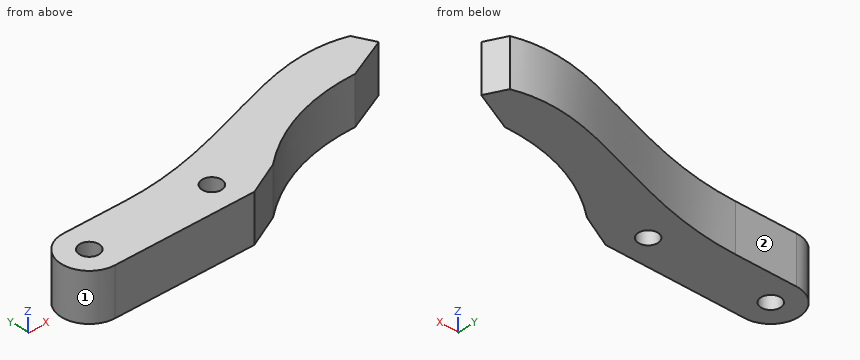
from build123d import *

# Parameters (mm, degrees)
SKETCH1_R           = 5
SKETCH1_R_2         = 1.75
BOSS_EXTRUDE1_DEPTH = 8.5
BOSS_EXTRUDE2_START = -8.5
BOSS_EXTRUDE2_DEPTH = 8.5


with BuildPart() as part:
    # Sketch1 → Boss-Extrude1 (new body)
    # profile 1 of 3: a face of its own
    with BuildSketch(Plane.XY):
        with Locations((-11, 0)):
            Circle(SKETCH1_R)
        with Locations((-11, 0)):
            Circle(SKETCH1_R_2, mode=Mode.SUBTRACT)
    # profile 2 of 3: a face of its own
    with BuildSketch(Plane.XY):
        with BuildLine():
            Line((11, 5), (-11, 5))
            ThreePointArc((-11, 5), (-7.464466094, 3.535533906), (-6, 0))
            ThreePointArc((-6, 0), (-7.464466094, -3.535533906), (-11, -5))
            Line((-11, -5), (11, -5))
            ThreePointArc((11, -5), (6, 0), (11, 5))
        make_face()
    # profile 3 of 3: a face of its own
    with BuildSketch(Plane.XY):
        with Locations((11, 0)):
            Circle(SKETCH1_R)
        with Locations((11, 0)):
            Circle(SKETCH1_R_2, mode=Mode.SUBTRACT)
    extrude(amount=BOSS_EXTRUDE1_DEPTH)

    # Sketch2 → Boss-Extrude2 (add)
    with BuildSketch(Plane.XY.offset(8.5).offset(BOSS_EXTRUDE2_START)):
        with BuildLine():
            Line((0, 5), (11, 5))
            ThreePointArc((11, 5), (16, 0), (11, -5))
            Line((11, -5), (13.99, -5))
            Line((13.99, -5), (20.08, -2.029708536))
            add(Edge.make_bspline(
                [(20.08, -2.029708536), (29.738723452, 6.188270814), (42.27, 6)],
                knots=[0, 0, 0, 1, 1, 1], degree=2))
            Line((42.27, 6), (49.557013712, 9.301428655))
            Line((49.557013712, 9.301428655), (47.75, 12.87))
            add(Edge.make_bspline(
                [(0, 5), (8.211836031, 5.003252827), (16.545155604, 7.403359581), (31.829335326, 12.436602795), (40.713583566, 15.205464732), (47.75, 12.87)],
                knots=[0, 0, 0, 0, 0.466100506, 0.566100506, 1, 1, 1, 1], degree=3))
        make_face()
    extrude(amount=BOSS_EXTRUDE2_DEPTH)


solid = part.part
Here's how the part is built. I have some questions about the finished solid (model axes, mm). Face numbers are marked on the shaded views. A direction names the side the tool comes from. Coordinates: 2 decimals unless noted, no trailing zeros. Order: outer loops, then holes, each group sorted by start corner. A loop starts at its lowest first (then second) coordinate and runs counter-clockwise, first axis right, second up. Notation, with made-up numbers: (42.25, 30.5) - (82.25, 30.5) arc R15 ccw to (82.25, 46.5) - close; hole circle Ø3 at (-5.75, -9.75). An arc over 180 degrees is marked (long way). Use CSV: the item, a comma, the result in double quotes. Start each with the question number.
1. For the marked faces 1 and 2, which set-ups out of +Z, -Z, +X, -X, +Y, -Y let a thin tool reach every point of the face, with its end or its side?
2. Suppose I cut it at B-B on x = -1. List the corners of the cut face in (y, z) for me, then the cut area to 3 significant figures.
3. Suppose I cut it at D-D on y = -3.5. List the corners of the cut face in (x, z) for me.
4. Please list where these lines run through material, in increasing order: line 1 (Y direction, x = -11, z = 4.5); line 2 (X direction, y = 0.25, z = 5.25); line 3 (X direction, y = 0.5, z = 6.5). Write a range as from..to.
5. Suppose I cut it at A-A on z = 7.5. Give the number of separate pieces and of enclosed holes in the cut face, then the cut area to 3 significant figures.
Output:
1,face 1,"+Z, -Z, -X"
1,face 2,"+Z, -Z, -X, +Y"
2,outline,"(-5, 0) - (5, 0) - (5, 8.5) - (-5, 8.5) - close"
2,area,"85.0 mm2"
3,outline,"(-14.57, 0) - (17.07, 0) - (17.07, 8.5) - (-14.57, 8.5) - close"
4,line 1,"y = -5..-1.75, 1.75..5"
4,line 2,"x = -15.99..-12.73, -9.27..9.27, 12.73..23.05"
4,line 3,"x = -15.97..-12.68, -9.32..9.32, 12.68..23.41"
5,separate pieces,"1"
5,enclosed holes,"2"
5,area,"569 mm2"
